Design review of the part built by this model. Coordinates are the model's own, in mm. A direction names the side the tool comes from. Round coordinates to 2 decimals unless told otherwise and drop trailing zeros. Write each loop counter-clockwise with the first axis right and the second up, starting at its lowest first coordinate (ties: lowest second). Pieces come first, ordered by that corner, then holes. Notation, with made-up numbers: (-34, 86.5) -> (21, 86.5) arc R30 cw to (21, 123.5) -> close; hole circle Ø9 at (65.25, -32). An arc over 180 degrees is marked (long way). One line per question, with ' | ' between items. Start each with the question number.
1) Mouldability with a two-part tool opening along X and no side actions: class faces 1 (the flat face through (0, 15, 50)), 2 (the flat face through (1.87, 11.83, -32.73)), 3 (the flat face through (-17, 0, 0)) as +X half, -X half, draft (parallel to the pull), parting line (faces both ways), or undercut.
2) Insertion check: pin 1 Ø8 at (x, z) = (-7, 13) entering from +Y; pin 2 Ø6 at (y, z) = (25, 40) entering from +X; pin 3 Ø1.2 at (y, z) = (15, -32.5) entering from -X. Each pin has a flat end and moves straight along its axis. Give the tip position at first contact, or say it passes through.
3) Consider section D-D (y = 25). Count the separate pieces of the cut face and the enclosed holes in it, then the cut area to 3 significant figures.
4) For probe 1 along X at (y, z) = (15.5, 5); probe 2 along X at (y, z) = (6.5, 8.5); probe 3 along Y at (x, z) = (18.05, 10.5), list the stretches that pass through material, from the lowest coordinate up.
5) Consider section C-C (z = 53.5). Give the boundary of the cut face in (x, y).
6) For faces 4 (the flat face through (-1.815, 11.798, -32.732)), 5 (the cylindrical face through (-6.691, 27.864, -0.399)), 6 (the cylindrical face through (-0.92, 19.15, -31.25)), list the 3-axis set-ups (+Z, -Z, +X, -X, +Y, -Y) from which the entire face can be reached by the end or side of a thin tool; tool diameter is ignored.
7) Consider section A-A (z = 10.5). Give the boundary of the cut face in (x, y), then the cut area to 3 significant figures.
8) Consider section B-B (z = -22.5). Give the boundary of the cut face in (x, y).
```python
from build123d import *

# Parameters (mm, degrees)
SKETCH1_W           = 38
SKETCH1_H           = 62
BOSS_EXTRUDE1_DEPTH = 30
SKETCH2_W           = 33
SKETCH2_H           = 57
CUT_EXTRUDE1_DEPTH  = 30
FILLET1_R           = 4
SKETCH3_R           = 1.5
CUT_EXTRUDE2_DEPTH  = 2.5
SKETCH4_R           = 14.5
BOSS_EXTRUDE2_DEPTH = 57
SKETCH5_R           = 4.25
BOSS_EXTRUDE3_DEPTH = 0.5
BOSS_EXTRUDE4_DEPTH = 2.5
SKETCH8_R           = 3.6
BOSS_EXTRUDE5_DEPTH = 4.5
FILLET2_R           = 2
SKETCH10_R          = 7.25
BOSS_EXTRUDE6_DEPTH = 16.5
SKETCH11_R          = 11.75
BOSS_EXTRUDE7_DEPTH = 1
SKETCH12_R          = 7.25
BOSS_EXTRUDE8_DEPTH = 15
SKETCH13_W          = 4.5
SKETCH13_H          = 14.5
CUT_EXTRUDE3_DEPTH  = 13.5
SKETCH15_R          = 15
BOSS_EXTRUDE9_DEPTH = 16.5
BOSS_EXTRUDE9_TAPER = 20


with BuildPart() as part:
    # Sketch1 → Boss-Extrude1 (new body)
    with BuildSketch(Plane(origin=(0, 0, 0), x_dir=(1, 0, 0), z_dir=(0, 1, 0))):
        Rectangle(SKETCH1_W, SKETCH1_H)
    extrude(amount=BOSS_EXTRUDE1_DEPTH)

    # Sketch2 → Cut-Extrude1 (cut)
    with BuildSketch(Plane(origin=(0, 30, 0), x_dir=(1, 0, 0), z_dir=(0, 1, 0))):
        Rectangle(SKETCH2_W, SKETCH2_H)
    extrude(amount=-CUT_EXTRUDE1_DEPTH, mode=Mode.SUBTRACT)

    # Fillet1
    fillet1_edges = [part.edges().sort_by_distance(p)[0] for p in [
        (-19, 15, -31),
        (19, 15, -31),
    ]]
    fillet(fillet1_edges, radius=FILLET1_R)

    # Sketch3 → Cut-Extrude2 (cut)
    with BuildSketch(Plane(origin=(19, 0, 0), x_dir=(0, 0, -1), z_dir=(1, 0, 0))):
        with Locations((17.5, 25)):
            Circle(SKETCH3_R)
        with Locations((17.5, 5)):
            Circle(SKETCH3_R)
        with Locations((-10.5, 25)):
            Circle(SKETCH3_R)
        with Locations((-10.5, 5)):
            Circle(SKETCH3_R)
    extrude(amount=-CUT_EXTRUDE2_DEPTH, mode=Mode.SUBTRACT)

    # Sketch4 → Boss-Extrude2 (add)
    with BuildSketch(Plane.XY.offset(-28.5)):
        with Locations(Location((0, 15, 0), (0, 0, 180))):
            Circle(SKETCH4_R)
    extrude(amount=BOSS_EXTRUDE2_DEPTH)

    # Sketch5 → Boss-Extrude3 (add)
    with BuildSketch(Plane(origin=(0, 0, -31), x_dir=(-1, 0, 0), z_dir=(0, 0, -1))):
        with Locations(Location((0, 15, 0), (0, 0, 180))):
            Circle(SKETCH5_R)
    extrude(amount=BOSS_EXTRUDE3_DEPTH)

    # Sketch6 → Boss-Extrude4 (add)
    with BuildSketch(Plane(origin=(0, 0, -31.5), x_dir=(-1, 0, 0), z_dir=(0, 0, -1))):
        Polygon((0, 19.25), (-3.680607966, 17.125), (-3.680607966, 12.875), (0, 10.75), (3.680607966, 12.875), (3.680607966, 17.125), align=None)
    extrude(amount=BOSS_EXTRUDE4_DEPTH)

    # Sketch8 → Boss-Extrude5 (add)
    with BuildSketch(Plane(origin=(0, 0, -34), x_dir=(-1, 0, 0), z_dir=(0, 0, -1))):
        with Locations((0, 15)):
            Circle(SKETCH8_R)
    extrude(amount=BOSS_EXTRUDE5_DEPTH)

    # Fillet2
    fillet2_edges = [part.edges().sort_by_distance(p)[0] for p in [
        (3.6, 15, -38.5),
    ]]
    fillet(fillet2_edges, radius=FILLET2_R)

    # Sketch10 → Boss-Extrude6 (add)
    with BuildSketch(Plane.XY.offset(31)):
        with Locations((0, 15)):
            Circle(SKETCH10_R)
    extrude(amount=BOSS_EXTRUDE6_DEPTH)

    # Sketch11 → Boss-Extrude7 (add)
    with BuildSketch(Plane.XY.offset(47.5)):
        with Locations((0, 15)):
            Circle(SKETCH11_R)
    extrude(amount=BOSS_EXTRUDE7_DEPTH)

    # Sketch12 → Boss-Extrude8 (add)
    with BuildSketch(Plane.XY.offset(48.5)):
        with Locations((0, 15)):
            Circle(SKETCH12_R)
    extrude(amount=BOSS_EXTRUDE8_DEPTH)

    # Sketch13 → Cut-Extrude3 (cut)
    with BuildSketch(Plane.XY.offset(63.5)):
        with Locations((0, 15)):
            Rectangle(SKETCH13_W, SKETCH13_H)
    extrude(amount=-CUT_EXTRUDE3_DEPTH, mode=Mode.SUBTRACT)

    # Sketch15 → Boss-Extrude9 (add)
    with BuildSketch(Plane.XY.offset(31)):
        with Locations((0, 15)):
            Circle(SKETCH15_R)
    extrude(amount=BOSS_EXTRUDE9_DEPTH, taper=BOSS_EXTRUDE9_TAPER)


solid = part.part
```
From the geometry:
1) face 1: undercut | face 2: +X half | face 3: draft
2) pin 1: stops at y = 29.19 | pin 2: stops at x = 9.79 | pin 3: stops at x = -3.68
3) separate pieces: 3 | enclosed holes: 1 | area: 1,860 mm2
4) probe 1: x = -19 to -16.5, -14.49 to 14.49, 16.5 to 19 | probe 2: x = -19 to -16.5, -11.75 to 11.75, 16.5 to 19 | probe 3: y = 0 to 3.5, 6.5 to 23.5, 26.5 to 30
5) outline: (-2.25, 8.11) -> (-2.25, 21.89) arc R7.25 ccw to start; (2.25, 8.11) arc R7.25 ccw to (2.25, 21.89) -> close
6) face 4: -Z, -X, -Y | face 5: none | face 6: -Z
7) outline: (-19, 0) -> (-16.5, 0) -> (-16.5, 30) -> (-19, 30) -> close; circle Ø29 at (0, 15); (16.5, 0) -> (19, 0) -> (19, 3.5) -> (16.5, 3.5) -> close; (16.5, 6.5) -> (19, 6.5) -> (19, 23.5) -> (16.5, 23.5) -> close; (16.5, 26.5) -> (19, 26.5) -> (19, 30) -> (16.5, 30) -> close | area: 796 mm2
8) outline: (-19, 0) -> (-16.5, 0) -> (-16.5, 30) -> (-19, 30) -> close; circle Ø29 at (0, 15); (16.5, 0) -> (19, 0) -> (19, 30) -> (16.5, 30) -> close
